Here's the drawing with two shaded views (mm, measured from the low corner). I have some questions. A direction names the side the tool comes from. Give positions to 0.01 mm unless a question says otherwise; leave off trailing zeros. Loops run counter-clockwise (first coordinate to the right, second up) from the corner with the lowest first, then second, coordinate; pieces in that order, holes last. Notation, with made-up numbers: (57, -33.75) -> (75, -33.75) arc R30 cw to (75, 3.25) -> close; hole circle Ø1 at (-33, -1.5). An arc over 180 degrees is marked (long way). Answer in a Markdown table with one row per item. Add a question column.
Item 1: If we section it at C-C (z = 250): Write out the boundary of the cut face in (x, y).
Item 2: If we section it at A-A (x = 600): Write out the boundary of the cut face in (y, z).
Item 3: If we section it at B-B (y = 128.5): Write out the boundary of the cut face in (x, z).
Item 4: If I drill on line 1 (Y direction, x = 628, z = 376.5); line 2 (Z direction, x = 600, y = 90); line 3 (X direction, y = 162, z = 284.5) (1 decimal), over which ranges is the centre line in solid material (lowest first)?
Item 5: Which directions (+Z, -Z, +X, -X, +Y, -Y) give clear straight access to the entire face, cutting with the end or side of a thin tool? Please do the marked faces 4 and 5.
Item 6: We'd pull the mould along Z, two halves only. Please class the marked faces 1, 2 and 3: released by +Z, released by -Z, zero draft, split by the parting line, or undercut.
Item 7: If we section it at D-D (x = 250): Write out the boundary of the cut face in (y, z).
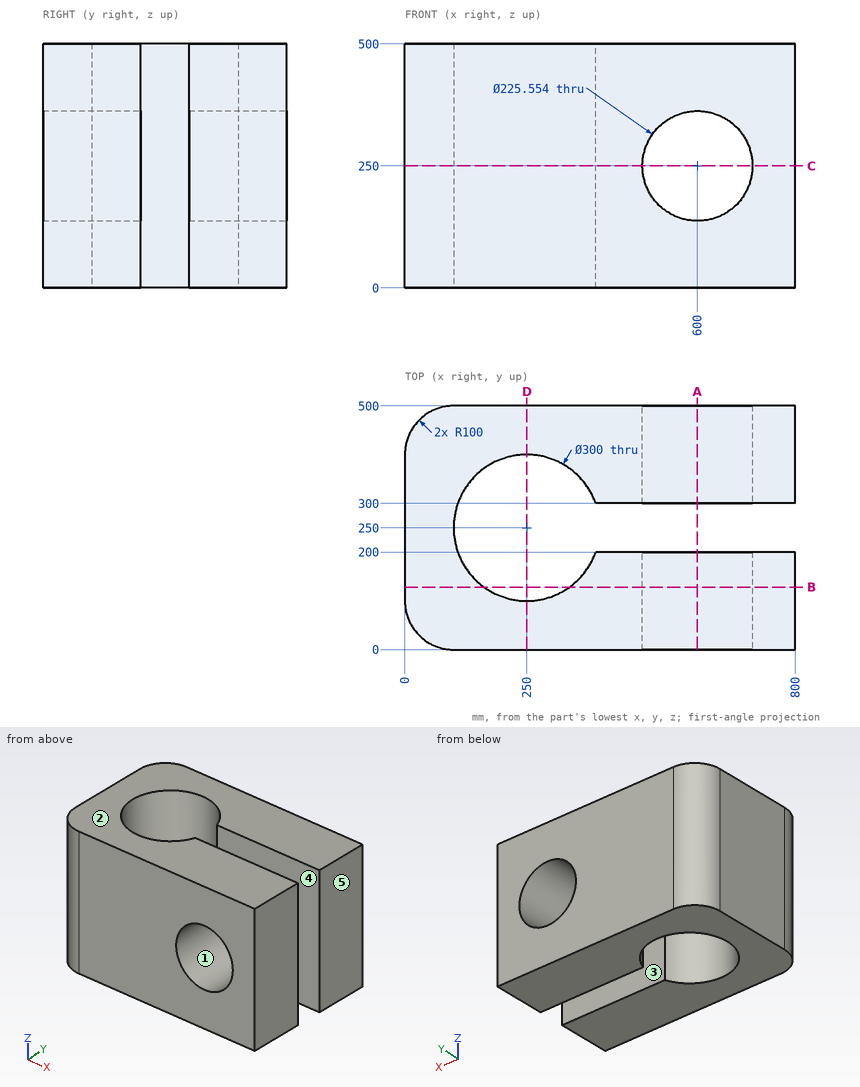
Recorded:
| question | item | result |
|---|---|---|
| 1 | outline | (0, 100) arc R100 ccw to (100, 0) -> (487.22, 0) -> (487.22, 200) -> (391.42, 200) arc R150 cw (long way) to (391.42, 300) -> (487.22, 300) -> (487.22, 500) -> (100, 500) arc R100 ccw to (0, 400) -> close; (712.78, 0) -> (800, 0) -> (800, 200) -> (712.78, 200) -> close; (712.78, 300) -> (800, 300) -> (800, 500) -> (712.78, 500) -> close |
| 2 | outline | (0, 0) -> (200, 0) -> (200, 137.22) -> (0, 137.22) -> close; (0, 362.78) -> (200, 362.78) -> (200, 500) -> (0, 500) -> close; (300, 0) -> (500, 0) -> (500, 137.22) -> (300, 137.22) -> close; (300, 362.78) -> (500, 362.78) -> (500, 500) -> (300, 500) -> close |
| 3 | outline | (0, 0) -> (162.04, 0) -> (162.04, 500) -> (0, 500) -> close; (337.96, 0) -> (800, 0) -> (800, 500) -> (337.96, 500) -> close; hole circle Ø225.55 at (600, 250) |
| 4 | line 1 | y = 0 to 200, 300 to 500 |
| 4 | line 2 | z = 0 to 137.22, 362.78 to 500 |
| 4 | line 3 | x = 0 to 128.5, 371.5 to 492.6, 707.4 to 800 |
| 5 | face 4 | +Z, -Z, +X |
| 5 | face 5 | +Z, -Z, +X, +Y, -Y |
| 6 | face 1 | undercut |
| 6 | face 2 | released by +Z |
| 6 | face 3 | zero draft |
| 7 | outline | (0, 0) -> (100, 0) -> (100, 500) -> (0, 500) -> close; (400, 0) -> (500, 0) -> (500, 500) -> (400, 500) -> close |
